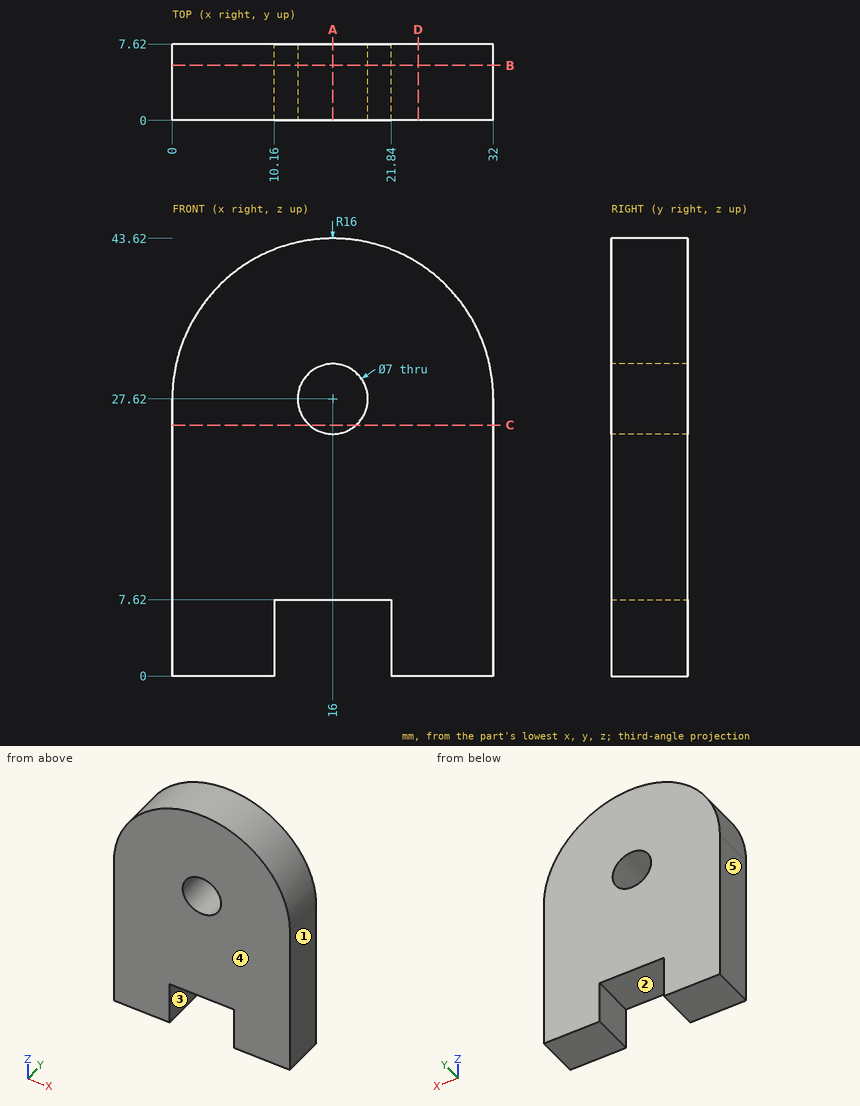
Study the drawing (mm; zero at the part's minimum x, y, z) and answer. A direction names the side the tool comes from. Give positions to 0.01 mm unless a question says otherwise; leave off trailing zeros. Order: outer loops, then holes, each group sorted by start corner. A loop starts at its lowest first (then second) coordinate and runs counter-clockwise, first axis right, second up. Notation, with made-up numbers: (51.5, 60.25) - (66.5, 60.25) arc R24 ccw to (66.5, 98.25) - close; hole circle Ø6 at (51.25, 76). An arc over 180 degrees is marked (long way). Answer as CSV lines item,"result". Start each with the question number.
Q1. The mould has two halves that part along X. Classify the marked faces 3, 4 and 5: +X half, -X half, draft (parallel to the pull), parting line (faces both ways), or undercut.
Q2. The part is cut by section A-A (x = 16). Write down the section's boundary in (y, z), then the cut area to 3 significant figures.
Q3. For the marked faces 1 and 2, determine the directions among +Z, -Z, +X, -X, +Y, -Y from which every point of the face is accessible in a straight line to the end or side of a thin tool.
Q4. Find the intervals of material crossed by L1, parallel to Z at x = 16, y = 5.5; L2, parallel to X at y = 3.25, z = 5; L3, parallel to Z at x = 17.5, y = 5.25, in increasing order. Write a range as [from, to].
Q5. Given pin 1 Ø2 at (x, y) = (24.5, 1) entering from +Z; pin 2 Ø1.5 at (x, y) = (9, 4) entering from -Z; pin 3 Ø2 at (y, z) = (6.5, 36.5) entering from +X (3 decimals), each flat-ended and moving along its own axis, determine where each tip first touches the part or whether it passes through.
Q6. The part is cut by section B-B (y = 5.5). Write down the section's boundary in (x, z), then the cut area to 3 significant figures.
Q7. The part is cut by section D-D (x = 24.5). Write down the section's boundary in (y, z).
Q8. The part is cut by section C-C (z = 25). Write down the section's boundary in (x, y).
Check result:
1,face 3,"undercut"
1,face 4,"draft"
1,face 5,"-X half"
2,outline,"(0, 7.62) - (7.62, 7.62) - (7.62, 24.12) - (0, 24.12) - close; (0, 31.12) - (7.62, 31.12) - (7.62, 43.62) - (0, 43.62) - close"
2,area,"221 mm²"
3,face 1,"+Z, -Z, +X, +Y, -Y"
3,face 2,"-Z, +Y, -Y"
4,L1,"z = [7.62, 24.12], [31.12, 43.62]"
4,L2,"x = [0, 10.16], [21.84, 32]"
4,L3,"z = [7.62, 24.46], [30.78, 43.55]"
5,pin 1,"stops at z = 41.75"
5,pin 2,"stops at z = 0"
5,pin 3,"stops at x = 29.925"
6,outline,"(0, 0) - (10.16, 0) - (10.16, 7.62) - (21.84, 7.62) - (21.84, 0) - (32, 0) - (32, 27.62) arc R16 ccw to (0, 27.62) - close; hole circle Ø7 at (16, 27.62)"
6,area,"1,160 mm²"
7,outline,"(0, 0) - (7.62, 0) - (7.62, 41.18) - (0, 41.18) - close"
8,outline,"(0, 0) - (13.68, 0) - (13.68, 7.62) - (0, 7.62) - close; (18.32, 0) - (32, 0) - (32, 7.62) - (18.32, 7.62) - close"
